from build123d import *

# Parameters (mm, degrees)
SKETCH1_W            = 63.5
SKETCH1_H            = 88.9
EXTRUDE1_DEPTH       = 12.192
SKETCH2_R            = 4.953
CUT_EXTRUDE1_DEPTH   = 13.192
LPATTERN1_COUNT      = 2
LPATTERN1_PITCH      = 63.5
LPATTERN1_COUNT_DIR2 = 2
LPATTERN1_PITCH_DIR2 = 38.1
FILLET1_R            = 12.7
EXTRUDE2_DEPTH       = 33.782
CUT_EXTRUDE3_DEPTH   = 74.683081323


with BuildPart() as part:
    # Sketch1 → Extrude1 (new body)
    with BuildSketch(Plane(origin=(0, 0, 0), x_dir=(1, 0, 0), z_dir=(0, 1, 0))):
        with Locations((2.085074627, -2.677425373)):
            Rectangle(SKETCH1_W, SKETCH1_H)
    extrude(amount=-EXTRUDE1_DEPTH)

    # Sketch2 → Cut-Extrude1 (cut, through all)
    with BuildSketch(Plane(origin=(0, 0, 0), x_dir=(-1, 0, 0), z_dir=(0, 1, 0))):
        with Locations((-21.135074627, 34.427425373)):
            Circle(SKETCH2_R)
    cut_extrude1 = extrude(amount=-CUT_EXTRUDE1_DEPTH, mode=Mode.SUBTRACT)

    # LPattern1: Cut-Extrude1 2 × 2
    with Locations(*[(-j * LPATTERN1_PITCH_DIR2, 0, -i * LPATTERN1_PITCH) for i in range(LPATTERN1_COUNT) for j in range(LPATTERN1_COUNT_DIR2) if (i, j) != (0, 0)]):
        add(cut_extrude1, mode=Mode.SUBTRACT)

    # Fillet1
    fillet1_edges = [part.edges().sort_by_distance(p)[0] for p in [
        (-29.664925373, -6.096, -41.772574627),
        (33.835074627, -6.096, -41.772574627),
        (33.835074627, -6.096, 47.127425373),
        (-29.664925373, -6.096, 47.127425373),
    ]]
    fillet(fillet1_edges, radius=FILLET1_R)

    # Sketch4 → Extrude2 (add)
    with BuildSketch(Plane(origin=(0, 0, 0), x_dir=(-1, 0, 0), z_dir=(0, 1, 0))):
        Polygon((-0.31333595, -25.325077129), (-22.53833595, 13.169752069), (4.95797062, 29.044752069), (27.18297062, -9.450077129), align=None)
    extrude(amount=EXTRUDE2_DEPTH)

    # Sketch5 → Cut-Extrude3 (cut, through all)
    with BuildSketch(Plane(origin=(11.337253914, 0, 19.636699798), x_dir=(0.866025404, 0, -0.5), z_dir=(0.5, 0, 0.866025404))):
        Polygon((-110.61611964, 175.14986028), (-15.514104542, 33.782), (-6.116104542, 19.812), (-6.116104542, 14.732), (0.233895458, 14.732), (0.233895458, 19.812), (9.631895458, 33.782), (104.733910555, 175.14986028), (104.733910555, 515.909395413), (-110.61611964, 515.909395413), align=None)
    extrude(amount=-CUT_EXTRUDE3_DEPTH, mode=Mode.SUBTRACT)


solid = part.part
Here's how the part is built. I have some questions about the finished solid (model axes, mm). A direction names the side the tool comes from. Coordinates: 2 decimals unless noted, no trailing zeros. Write each loop counter-clockwise with the first axis right and the second up, starting at its lowest first coordinate (ties: lowest second). Pieces come first, ordered by that corner, then holes. Notation, with made-up numbers: (56, -3) - (102, -3) arc R21 ccw to (102, 18) - close; hole circle Ø3 at (29, -24). An arc over 180 degrees is marked (long way). Use one line per item in the form item = value.
1) I'm going to push flat-ended pins straight in: P1, Ø1, axis at y = 5.5, z = -5.5, coming from the +X side; P2, Ø6, axis at y = 14, z = -15, coming from the -X side; P3, Ø1, axis at y = 27, z = -20.5, coming from the +X side. Where does each tip first touch, or does it pass through?
Solved:
P1 = 12.05
P2 = -22.77
P3 = 3.39
2) Suppose I cut it at D-D, the plane y = 30.5. Write out the boundary of the cut face in (x, z).
Solved:
outline = (-27.18, -9.45) - (-22.41, -12.21) - (-0.19, 26.29) - (-4.96, 29.04) - close; (-4.46, -22.57) - (0.31, -25.33) - (22.54, 13.17) - (17.77, 15.92) - close
3) Suppose I cut it at B-B, the plane z = -26.5. Write out the boundary of the cut face in (x, y).
Solved:
outline = (-29.66, -12.19) - (-21.2, -12.19) - (-21.2, 0) - (-29.66, 0) - close; (-12.73, -12.19) - (16.9, -12.19) - (16.9, 0) - (-12.73, 0) - close; (25.37, -12.19) - (33.84, -12.19) - (33.84, 0) - (25.37, 0) - close
4) Suppose I cut it at A-A, the plane y = -6. Write out the boundary of the cut face in (x, z), plus the area to 3 significant figures.
Solved:
outline = (-29.66, -29.07) arc R12.7 ccw to (-16.96, -41.77) - (21.14, -41.77) arc R12.7 ccw to (33.84, -29.07) - (33.84, 34.43) arc R12.7 ccw to (21.14, 47.13) - (-16.96, 47.13) arc R12.7 ccw to (-29.66, 34.43) - close; hole circle Ø9.91 at (-16.96, -29.07); hole circle Ø9.91 at (-16.96, 34.43); hole circle Ø9.91 at (21.14, -29.07); hole circle Ø9.91 at (21.14, 34.43)
area = 5,200 mm2
5) Thinking about a two-plate mould opening in Z: for faces 6 (the cylindrical face through (16.56, -6.01, 32.53)), 7 (the flat face through (0.58, 17.24, 0.54)), 8 (the flat face through (11.27, 16.65, -6.35)), 9 (the cylindrical face through (-26.04, -6.18, 43.31)), which applies, released by +Z, released by -Z, zero draft, split by the parting line, or undercut?
Solved:
face_6 = undercut
face_7 = undercut
face_8 = released by -Z
face_9 = released by +Z
6) Suppose I cut it at C-C, the plane x = -19. Write out the boundary of the cut face in (y, z).
Solved:
outline = (-12.19, -41.61) - (0, -41.61) - (0, -33.59) - (-12.19, -33.59) - close; (-12.19, -24.56) - (0, -24.56) - (0, -14.17) - (24.64, -14.17) - (33.78, -1.88) - (33.78, 4.72) - (0, 4.72) - (0, 29.91) - (-12.19, 29.91) - close; (-12.19, 38.94) - (0, 38.94) - (0, 46.96) - (-12.19, 46.96) - close
7) I need wall thicknesses on line 1 (Y direction, x = 4.5, z = -24); line 2 (X direction, y = 23.5, z = 16); line 3 (X direction, y = 21, z = -1.5). Which ranges of each line are inside material? Lowest first, please.
Solved:
line_1 = -12.19 to 0
line_2 = -12.49 to -0.69, 12.37 to 17.64
line_3 = -22.59 to -8.85, 0.33 to 14.07
8) On a 3-axis mill with a long thin cutter (end or side, diameter ignored), from which of +Z, -Z, +X, -X, +Y, -Y can I reach the whole of each face in a straight line? I mean faces 1 (the flat face through (16, 0, -8)), 2 (the flat face through (-13.627, 12.901, -17.276)), 3 (the flat face through (-15.915, 16.655, 10.067)), 4 (the cylindrical face through (30.016, -6.181, 43.506)), 5 (the cylindrical face through (30.016, -6.181, -38.151)). Say none if no direction works.
Solved:
face_1 = +Y
face_2 = -Z, -X, +Y
face_3 = +Z, -X, +Y
face_4 = +Z, +X, +Y, -Y
face_5 = -Z, +X, +Y, -Y
